```python
from build123d import *

# Parameters (mm, degrees)
F0_R     = 28.575
F0_R_2   = 11
F1_DEPTH = 9.525
F3_DEPTH = 25.4
F4_R     = 2.38125
F5_DEPTH = 25.4
F6_R     = 2


with BuildPart() as f1:
    # F0 (on Top) → F1 (new body)
    with BuildSketch(Plane.XY):
        Circle(F0_R)
        Circle(F0_R_2, mode=Mode.SUBTRACT)
    extrude(amount=F1_DEPTH)

    # F2 (on Top) → F3 (cut)
    with BuildSketch(Plane.XY):
        with BuildLine():
            ThreePointArc((6.6033751745, -33.3637991738), (17.0054966041, -29.4543841262), (25.592210064, -22.4005902387))
            ThreePointArc((25.592210064, -22.4005902387), (11.4492466041, -19.8306768266), (6.6033751745, -33.3637991738))
        make_face()
        with BuildLine():
            ThreePointArc((-25.592210064, -22.4005902387), (-17.0054966041, -29.4543841262), (-6.6033751745, -33.3637991738))
            ThreePointArc((-6.6033751745, -33.3637991738), (-6.0720335059, -31.4411002438), (-5.8929966041, -29.4543841262))
            ThreePointArc((-5.8929966041, -29.4543841262), (-13.259311683, -18.9923692731), (-25.592210064, -22.4005902387))
        make_face()
        with BuildLine():
            ThreePointArc((-22.8984932081, 0), (-25.5356944726, 7.187278177), (-32.1955852385, 10.9632089351))
            ThreePointArc((-32.1955852385, 10.9632089351), (-34.0109932081, 0), (-32.1955852385, -10.9632089351))
            ThreePointArc((-32.1955852385, -10.9632089351), (-25.5356944726, -7.187278177), (-22.8984932081, 0))
        make_face()
        with BuildLine():
            ThreePointArc((-5.8929966041, 29.4543841262), (-6.0720335059, 31.4411002438), (-6.6033751745, 33.3637991738))
            ThreePointArc((-6.6033751745, 33.3637991738), (-17.0054966041, 29.4543841262), (-25.592210064, 22.4005902387))
            ThreePointArc((-25.592210064, 22.4005902387), (-13.259311683, 18.9923692731), (-5.8929966041, 29.4543841262))
        make_face()
        with BuildLine():
            ThreePointArc((6.6033751745, 33.3637991738), (11.4492466041, 19.8306768266), (25.592210064, 22.4005902387))
            ThreePointArc((25.592210064, 22.4005902387), (17.0054966041, 29.4543841262), (6.6033751745, 33.3637991738))
        make_face()
        with BuildLine():
            ThreePointArc((32.1955852385, -10.9632089351), (33.5540719577, -5.55625), (34.0109932081, 0))
            ThreePointArc((34.0109932081, 0), (33.5540719577, 5.55625), (32.1955852385, 10.9632089351))
            ThreePointArc((32.1955852385, 10.9632089351), (22.8984932081, 0), (32.1955852385, -10.9632089351))
        make_face()
    extrude(amount=F3_DEPTH, mode=Mode.SUBTRACT)

    # F4 (on Top) → F5 (cut)
    with BuildSketch(Plane.XY):
        with Locations((0, 22.86)):
            Circle(F4_R)
        with Locations((-19.7973407305, 11.43)):
            Circle(F4_R)
        with Locations((-19.7973407305, -11.43)):
            Circle(F4_R)
        with Locations((0, -22.86)):
            Circle(F4_R)
        with Locations((19.7973407305, -11.43)):
            Circle(F4_R)
        with Locations((19.7973407305, 11.43)):
            Circle(F4_R)
    extrude(amount=F5_DEPTH, mode=Mode.SUBTRACT)

    # F6
    f6_edges = [f1.edges().sort_by_distance(p)[0] for p in [
        (-5.996854, -27.938654, 4.7625),
        (-21.197157, -19.162755, 4.7625),
        (-27.194011, -8.775899, 4.7625),
        (-27.194011, 8.775899, 4.7625),
        (-21.197157, 19.162755, 4.7625),
        (-5.996854, 27.938654, 4.7625),
        (21.197157, 19.162755, 4.7625),
        (5.996854, 27.938654, 4.7625),
        (27.194011, 8.775899, 4.7625),
        (27.194011, -8.775899, 4.7625),
        (21.197157, -19.162755, 4.7625),
        (5.996854, -27.938654, 4.7625),
    ]]
    fillet(f6_edges, radius=F6_R)


solid = f1.part
```
Geometry: final body of the model. Coordinates: model frame, mm. Round coordinates to 2 decimals unless told otherwise and drop trailing zeros. Write each loop counter-clockwise with the first axis right and the second up, starting at its lowest first coordinate (ties: lowest second). Pieces come first, ordered by that corner, then holes.
Item 1: Section query B-B (x = 1). Return loops of the section in (y, z) (1 decimal).
Item 2: Section query C-C (y = -22). Return loops of the section in (x, z) (3 decimals), plus the area to 3 significant figures.
Item 3: Section query A-A (y = 22.86). Return loops of the section in (x, z) (3 decimals).
Item 4: Section query D-D (x = -12). Return loops of the section in (y, z) (3 decimals).
Item 5: Material intervals for L1, parallel to Y at x = 0, z = 2.75 (3 decimals); L2, parallel to X at y = -11.43, z = 7; L3, parallel to Y at x = 20, z = 2, sorted ascending.
Item 6: Pin query (flat end, axial travel): P1, Ø2, axis at y = 6, z = 7, coming from the +X side; P2, Ø4, axis at x = 3, z = 6.5, coming from the +Y side; P3, Ø5, axis at y = 5.5, z = 8, coming from the +X side. Return the tip coordinate at first contact, or that it passes through.
Completed:
1. outline: (-28.6, 0) - (-25, 0) - (-25, 9.5) - (-28.6, 9.5) - close; (-20.7, 0) - (-11, 0) - (-11, 9.5) - (-20.7, 9.5) - close; (11, 0) - (20.7, 0) - (20.7, 9.5) - (11, 9.5) - close; (25, 0) - (28.6, 0) - (28.6, 9.5) - (25, 9.5) - close
2. outline: (-8.764, 0) - (-2.221, 0) - (-2.221, 9.525) - (-8.764, 9.525) - close; (2.221, 0) - (8.764, 0) - (8.764, 9.525) - (2.221, 9.525) - close
2. area: 125 mm2
3. outline: (-8.061, 0) - (-2.381, 0) - (-2.381, 9.525) - (-8.061, 9.525) - close; (2.381, 0) - (8.061, 0) - (8.061, 9.525) - (2.381, 9.525) - close
4. outline: (-19.533, 0) - (19.533, 0) - (19.533, 9.525) - (-19.533, 9.525) - close
5. L1: y = -28.575 to -25.241, -20.479 to -11, 11 to 20.479, 25.241 to 28.575
5. L2: x = -26.19 to -22.18, -17.42 to 17.42, 22.18 to 26.19
5. L3: y = -18.75 to -13.8, -9.06 to 9.06, 13.8 to 18.75
6. P1: stops at x = 25.38
6. P2: stops at y = 28.56
6. P3: stops at x = 26.3
